```python
from build123d import *

# Parameters (mm, degrees)
ESBO_O1_R                = 1.5
RESSALTO_EXTRUS_O1_DEPTH = 3


with BuildPart() as part:
    # Esboço1 → Ressalto-extrusão1 (new body)
    with BuildSketch(Plane.XY):
        Polygon((40.700385396, -30.0684829), (10.700385396, -30.0684829), (10.700385396, -33.0684829), (-19.299614604, -33.0684829), (-19.299614604, -30.0684829), (-49.299614604, -30.0684829), (-49.299614604, -33.0684829), (-79.299614604, -33.0684829), (-79.299614604, -30.0684829), (-82.299614604, -30.0684829), (-82.299614604, -18.0684829), (-79.299614604, -18.0684829), (-79.299614604, -6.178045813), (-82.299614604, -6.178045813), (-82.299614604, 5.821954187), (-79.299614604, 5.821954187), (-79.299614604, 17.9315171), (-82.299614604, 17.9315171), (-82.299614604, 29.9315171), (-79.299614604, 29.9315171), (-79.299614604, 33), (-49.299614604, 33), (-49.299614604, 30), (-19.299614604, 30), (-19.299614604, 33), (10.700385396, 33), (10.700385396, 30), (40.700385396, 30), (40.700385396, 33), (70.700385396, 33), (70.700385396, 29.9315171), (73.700385396, 29.9315171), (73.700385396, 17.9315171), (70.700385396, 17.9315171), (70.700385396, 5.999991894), (73.700385396, 5.999991894), (73.700385396, -6.000008106), (70.700385396, -6.000008106), (70.700385396, -18.000008106), (73.700385396, -18.000008106), (73.700385396, -30.000008106), (70.700385396, -30.000008106), (70.700385396, -33.0684829), (40.700385396, -33.0684829), align=None)
        with Locations((33.200385396, 15)):
            Circle(ESBO_O1_R, mode=Mode.SUBTRACT)
        with Locations((-4.299614604, -0.178045813)):
            Circle(ESBO_O1_R, mode=Mode.SUBTRACT)
        with Locations((-41.799614604, 15)):
            Circle(ESBO_O1_R, mode=Mode.SUBTRACT)
        with Locations((-41.799614604, -0.178045813)):
            Circle(ESBO_O1_R, mode=Mode.SUBTRACT)
        with Locations((-4.299614604, -15.178045813)):
            Circle(ESBO_O1_R, mode=Mode.SUBTRACT)
        with Locations((-41.799614604, -15.178045813)):
            Circle(ESBO_O1_R, mode=Mode.SUBTRACT)
        with Locations((33.200385396, -0.178045813)):
            Circle(ESBO_O1_R, mode=Mode.SUBTRACT)
        with Locations((33.200385396, -15.178045813)):
            Circle(ESBO_O1_R, mode=Mode.SUBTRACT)
        with Locations((-4.299614604, 15)):
            Circle(ESBO_O1_R, mode=Mode.SUBTRACT)
    extrude(amount=RESSALTO_EXTRUS_O1_DEPTH)


solid = part.part
```
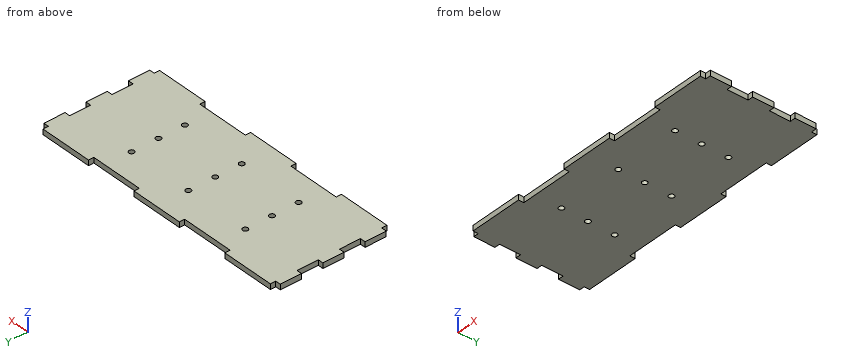
Verification items for the finished model (mm, model axes). Give positions to 0.01 mm unless a question says otherwise; leave off trailing zeros. Loops run counter-clockwise (first coordinate to the right, second up) from the corner with the lowest first, then second, coordinate; pieces in that order, holes last.
1. Section check A-A, the plane y = 15. Enter the section's corners in (x, z).
2. Section check B-B, the plane x = 24. Enter the section's corners in (y, z), then the cut area to 3 significant figures.
3. Go/stop test with flat-tipped pins: pin 1 Ø1 at (x, z) = (19, 2.5) entering from +Y; pin 2 Ø0.9 at (x, z) = (-80.5, 2) entering from -Y; pin 3 Ø1.5 at (y, z) = (-31, 2) entering from -X. Record where each tip stops, or that it passes through.
4. Section check D-D, the plane z = 0.55. Count the separate pieces of the cut face and the enclosed holes in it, then the cut area to 3 significant figures.
5. Thickness scan on line 1 (Y direction, x = 32, z = 1.65); line 2 (X direction, y = -16.5, z = 2.55); line 3 (Y direction, x = 40.5, z = 0.7). Record the ranges inside material, lowest first.
6. Section check C-C, the plane y = 8. Enter the section's corners in (x, z).
Geometry says:
1. outline: (-79.3, 0) - (-43.3, 0) - (-43.3, 3) - (-79.3, 3) - close; (-40.3, 0) - (-5.8, 0) - (-5.8, 3) - (-40.3, 3) - close; (-2.8, 0) - (31.7, 0) - (31.7, 3) - (-2.8, 3) - close; (34.7, 0) - (70.7, 0) - (70.7, 3) - (34.7, 3) - close
2. outline: (-30.07, 0) - (30, 0) - (30, 3) - (-30.07, 3) - close
2. area: 180 mm2
3. pin 1: stops at y = 30
3. pin 2: stops at y = -30.07
3. pin 3: stops at x = -79.3
4. separate pieces: 1
4. enclosed holes: 9
4. area: 9,700 mm2
5. line 1: y = -30.07 to -16.08, -14.28 to -1.08, 0.72 to 14.1, 15.9 to 30
5. line 2: x = -79.3 to -42.51, -41.09 to -5.01, -3.59 to 32.49, 33.91 to 70.7
5. line 3: y = -30.07 to 30
6. outline: (-79.3, 0) - (70.7, 0) - (70.7, 3) - (-79.3, 3) - close
